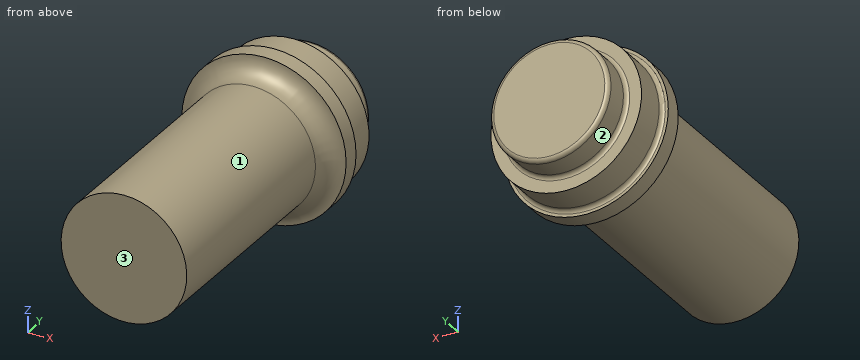
from build123d import *

# Parameters (mm, degrees)
SKETCH1_R           = 15.9
BOSS_EXTRUDE1_DEPTH = 62
SKETCH2_R           = 20.8
BOSS_EXTRUDE2_DEPTH = 4.4
SKETCH3_R           = 19.05
BOSS_EXTRUDE3_DEPTH = 8.8
SKETCH4_R           = 15.05
BOSS_EXTRUDE4_DEPTH = 7.5
FILLET1_R           = 5
FILLET2_R           = 1


with BuildPart() as part:
    # Sketch1 → Boss-Extrude1 (new body)
    with BuildSketch(Plane(origin=(0, 0, 0), x_dir=(1, 0, 0), z_dir=(0, 1, 0))):
        with Locations(Location((0, 0, 0), (0, 0, 270))):
            Circle(SKETCH1_R)
    extrude(amount=BOSS_EXTRUDE1_DEPTH)

    # Sketch2 → Boss-Extrude2 (add)
    with BuildSketch(Plane(origin=(0, 62, 0), x_dir=(1, 0, 0), z_dir=(0, 1, 0))):
        with Locations(Location((0, 0, 0), (0, 0, 270))):
            Circle(SKETCH2_R)
    extrude(amount=BOSS_EXTRUDE2_DEPTH)

    # Sketch3 → Boss-Extrude3 (add)
    with BuildSketch(Plane(origin=(0, 66.4, 0), x_dir=(1, 0, 0), z_dir=(0, 1, 0))):
        with Locations(Location((0, 0, 0), (0, 0, 270))):
            Circle(SKETCH3_R)
    extrude(amount=BOSS_EXTRUDE3_DEPTH)

    # Sketch4 → Boss-Extrude4 (add)
    with BuildSketch(Plane(origin=(0, 75.2, 0), x_dir=(1, 0, 0), z_dir=(0, 1, 0))):
        with Locations(Location((0, 0, 0), (0, 0, 270))):
            Circle(SKETCH4_R)
    extrude(amount=BOSS_EXTRUDE4_DEPTH)

    # Fillet1
    # the kernel refuses this fillet: 5 mm, written as the material it adds along each edge
    with BuildSketch(Plane(origin=(0, 62, 0), x_dir=(0, 0, 1), z_dir=(-1, 0, 0))) as fillet1_piece_1_section:
        with BuildLine():
            CenterArc((15.9 + FILLET1_R, -FILLET1_R), FILLET1_R, 90, 90)
            Line((15.9, -FILLET1_R), (15.9, 0))
            Line((15.9, 0), (15.9 + FILLET1_R, 0))
        make_face()
    fillet1_piece_1 = revolve(axis=Axis((0, 62, 0), (0, 1, 0)), mode=Mode.PRIVATE)
    fillet1_piece_1 = fillet1_piece_1 & Plane(origin=(0, 60.561583107, 0), x_dir=(0, 0, 1), z_dir=(0, -1, 0)) * Cylinder(20.8, 84, mode=Mode.PRIVATE)
    add(fillet1_piece_1)

    # Fillet2
    fillet2_edges = [part.edges().sort_by_distance(p)[0] for p in [
        (0, 75.2, -15.05),
        (0, 82.7, -15.05),
        (0, 66.4, -19.05),
    ]]
    fillet(fillet2_edges, radius=FILLET2_R)


solid = part.part
Geometry: final body of the model. Coordinates: model frame, mm. Face numbers are marked on the shaded views. A direction names the side the tool comes from. Round coordinates to 2 decimals unless told otherwise and drop trailing zeros. Loops run counter-clockwise (first coordinate to the right, second up) from the corner with the lowest first, then second, coordinate; pieces in that order, holes last. Notation, with made-up numbers: (57, 58) - (97, 58) arc R13 cw to (97, 68) - close; hole circle Ø7 at (74.5, -34.5). An arc over 180 degrees is marked (long way). Write each question's results on one line, items separated by ' | '. Start each with the question number.
1) Cut plane C-C on y = 63. Return loops of the section in (x, z).
2) Cut plane B-B on z = 0. Return loops of the section in (x, y).
3) Access query for the marked faces 1, 2 and 3. Directions: +Z, -Z, +X, -X, +Y, -Y. A direction counts if a zero-diameter tool reaches every point of the face in a straight line with its end or side. Return the directions, or none.
4) Cut plane A-A on x = 0. Return loops of the section in (y, z).
5) Cut plane D-D on y = 78. Return loops of the section in (x, z), then the cut area to 3 significant figures.
6) Line query: probe 1 along Z at (x, y) = (-0.5, 56); probe 2 along Y at (x, z) = (-1.5, -16.5); probe 3 along X at (y, z) = (41, 11.5). Output: solid intervals per line, ascending. Write a range as [from, to].
7) First-contact query: P1, Ø8, axis at y = 50.5, z = 4, coming from the -X side; P2, Ø12, axis at x = 0.5, y = 43.5, coming from the +Z side; P3, Ø3, axis at y = 9.5, z = 1, coming from the +X side. Flat tips, straight axial feed; report the tip coordinate or a pass-through.
Verdict:
1) outline: circle Ø41.6 at (0, 0)
2) outline: (-20.8, 62) arc R5 cw to (-15.9, 57) - (-15.9, 0) - (15.9, 0) - (15.9, 57) arc R5 cw to (20.8, 62) - (20.8, 66.4) - (20.05, 66.4) arc R1 cw to (19.05, 67.4) - (19.05, 75.2) - (16.05, 75.2) arc R1 cw to (15.05, 76.2) - (15.05, 81.7) arc R1 ccw to (14.05, 82.7) - (-14.05, 82.7) arc R1 ccw to (-15.05, 81.7) - (-15.05, 76.2) arc R1 cw to (-16.05, 75.2) - (-19.05, 75.2) - (-19.05, 67.4) arc R1 cw to (-20.05, 66.4) - (-20.8, 66.4) - close
3) face 1: -Y | face 2: +Y | face 3: +Z, -Z, +X, -X, -Y
4) outline: (0, -15.9) - (57, -15.9) arc R5 cw to (62, -20.8) - (66.4, -20.8) - (66.4, -20.05) arc R1 cw to (67.4, -19.05) - (75.2, -19.05) - (75.2, -16.05) arc R1 cw to (76.2, -15.05) - (81.7, -15.05) arc R1 ccw to (82.7, -14.05) - (82.7, 14.05) arc R1 ccw to (81.7, 15.05) - (76.2, 15.05) arc R1 cw to (75.2, 16.05) - (75.2, 19.05) - (67.4, 19.05) arc R1 cw to (66.4, 20.05) - (66.4, 20.8) - (62, 20.8) arc R5 cw to (57, 15.9) - (0, 15.9) - close
5) outline: circle Ø30.1 at (0, 0) | area: 712 mm2
6) probe 1: z = [-15.89, 15.89] | probe 2: y = [59.5, 75.2] | probe 3: x = [-10.98, 10.98]
7) P1: stops at x = -15.9 | P2: stops at z = 15.9 | P3: stops at x = 15.9
